```python
from build123d import *

# Parameters (mm, degrees)
F0_W      = 85.09
F0_H      = 165.1
F1_DEPTH  = 25.4
F2_W      = 39.37
F2_H      = 161.925
F3_DEPTH  = 22.225
F4_W      = 50.8
F4_H      = 5.08
F5_DEPTH  = 6.35
F7_DEPTH  = 25.401
F8_W      = 39.37
F8_H      = 15.24
F9_DEPTH  = 3.175
F10_W     = 6.35
F10_H     = 25.4
F11_DEPTH = 3.175
F12_R     = 5.08


with BuildPart() as f1:
    # F0 (on Top) → F1 (new body)
    with BuildSketch(Plane.XY):
        with Locations((-2.9836203903, 38.1636999707)):
            Rectangle(F0_W, F0_H)
    extrude(amount=F1_DEPTH)

    # F2 (on face) → F3 (cut)
    with BuildSketch(Plane.XY.offset(25.4)):
        with Locations((16.7013796097, 39.7511999707)):
            Rectangle(F2_W, F2_H)
    extrude(amount=-F3_DEPTH, mode=Mode.SUBTRACT)

    # F4 (on face) → F5 (join)
    with BuildSketch(Plane(origin=(36.3863796097, 0, 0), x_dir=(0, -1, 0), z_dir=(-1, 0, 0))):
        with Locations((-85.7886999707, 10.795)):
            Rectangle(F4_W, F4_H)
    extrude(amount=F5_DEPTH)

    # F6 (on face) → F7 (cut, through all)
    with BuildSketch(Plane.XY.offset(25.4)):
        Polygon((-2.9836203903, -41.2113000293), (-2.9836203903, 120.7136999707), (-45.5286203903, 120.7136999707), (-45.5286203903, -44.3863000293), (-2.9836203903, -44.3863000293), align=None)
    extrude(amount=-F7_DEPTH, mode=Mode.SUBTRACT)

    # F8 (on face) → F9 (join)
    with BuildSketch(Plane.XY.offset(25.4)):
        with Locations((16.7013796097, -33.5913000293)):
            Rectangle(F8_W, F8_H)
    extrude(amount=-F9_DEPTH)

    # F10 (on face) → F11 (join)
    with BuildSketch(Plane.XY.offset(3.175)):
        with Locations((-6.1586203903, 82.6136999707)):
            Rectangle(F10_W, F10_H)
        with Locations((-6.1586203903, 31.8136999707)):
            Rectangle(F10_W, F10_H)
        with Locations((-6.1586203903, -18.9863000293)):
            Rectangle(F10_W, F10_H)
    extrude(amount=-F11_DEPTH)

    # F12
    f12_edges = [f1.edges().sort_by_distance(p)[0] for p in [
        (39.56138, -44.3863, 12.7),
    ]]
    fillet(f12_edges, radius=F12_R)


solid = f1.part
```
Can you work these out from the model? Positions are in its coordinate system, mm. A direction names the side the tool comes from. Give positions to 0.01 mm unless a question says otherwise; leave off trailing zeros. Write each loop counter-clockwise with the first axis right and the second up, starting at its lowest first coordinate (ties: lowest second). Pieces come first, ordered by that corner, then holes. Notation, with made-up numbers: (63.5, -10.75) -> (77.5, -10.75) arc R23 ccw to (77.5, 20.25) -> close; hole circle Ø6 at (58.25, 88). An arc over 180 degrees is marked (long way). One line per item, written item: value.
Q1. For P1, Ø2.5, axis at x = -5, z = 2.5, coming from the +Y side; P2, Ø2.5, axis at x = -5, z = 2, coming from the -Y side; P3, Ø10, axis at x = 17.5, z = 15, coming from the +Y side; P4, Ø1.5, axis at x = -4, z = 22, coming from the -Y side, each with a flat end and sliding along its axis, tell me the tip position at first contact or that it passes through.
Results found:
P1: stops at y = 95.31
P2: stops at y = -31.69
P3: stops at y = -41.21
P4: passes through
Q2. Which directions (+Z, -Z, +X, -X, +Y, -Y) give clear straight access to the entire face, cutting with the end or side of a thin tool? Please do faces 1 (the face through (-2.984, 57, 2)), 2 (the face through (33, 60.389, 11)), 3 (the face through (33, 86, 8.255)).
Results found:
face 1: +Z, -Z, -X
face 2: +Z, -X
face 3: -X, +Y
Q3. Imagine slicing it at C-C on x = -4.5. Please give me the cut outline in (y, z) (3 decimals), and give its area (3 significant figures).
Results found:
outline: (-31.686, 0) -> (-6.286, 0) -> (-6.286, 3.175) -> (-31.686, 3.175) -> close; (19.114, 0) -> (44.514, 0) -> (44.514, 3.175) -> (19.114, 3.175) -> close; (69.914, 0) -> (95.314, 0) -> (95.314, 3.175) -> (69.914, 3.175) -> close
area: 242 mm^2
Q4. Imagine slicing it at D-D on x = 5.5. Please give me the cut outline in (y, z) (3 decimals), and give its area (3 significant figures).
Results found:
outline: (-44.386, 0) -> (120.714, 0) -> (120.714, 3.175) -> (-41.211, 3.175) -> (-41.211, 22.225) -> (-25.971, 22.225) -> (-25.971, 25.4) -> (-44.386, 25.4) -> close
area: 643 mm^2
Q5. We'd pull the mould along Z, two halves only. Please class faces 4 (the face through (13, 41, 3.175)), 5 (the face through (33, 86, 13.335)), 6 (the face through (16, -33, 22.225)), 7 (the face through (-2.984, -41.4, 13.7)): +Z half, -Z half, draft (parallel to the pull), parting line (faces both ways), or undercut.
Results found:
face 4: undercut
face 5: +Z half
face 6: undercut
face 7: draft
Q6. Imagine slicing it at A-A on x = 32.5. Please give me the cut outline in (y, z) (3 decimals).
Results found:
outline: (-44.386, 0) -> (120.714, 0) -> (120.714, 3.175) -> (-41.211, 3.175) -> (-41.211, 22.225) -> (-25.971, 22.225) -> (-25.971, 25.4) -> (-44.386, 25.4) -> close; (60.389, 8.255) -> (111.189, 8.255) -> (111.189, 13.335) -> (60.389, 13.335) -> close
Q7. Imagine slicing it at B-B on y = 89. Please give me the cut outline in (x, z) (3 decimals).
Results found:
outline: (-9.334, 0) -> (39.561, 0) -> (39.561, 25.4) -> (36.386, 25.4) -> (36.386, 13.335) -> (30.036, 13.335) -> (30.036, 8.255) -> (36.386, 8.255) -> (36.386, 3.175) -> (-9.334, 3.175) -> close
Q8. Please list where these lines run through material, in increasing order: line 1 (Z direction, x = 31.5, y = -34.5) (3 decimals); line 2 (Y direction, x = 8.5, z = 10.25); line 3 (Z direction, x = 35, y = 59) (3 decimals). Write a range as [from, to].
Results found:
line 1: z = [0, 3.175], [22.225, 25.4]
line 2: y = [-44.39, -41.21]
line 3: z = [0, 3.175]
